Geometry: final body of the model. Coordinates: model frame, mm. A direction names the side the tool comes from. Give positions to 0.01 mm unless a question says otherwise; leave off trailing zeros. Order: outer loops, then holes, each group sorted by start corner. A loop starts at its lowest first (then second) coordinate and runs counter-clockwise, first axis right, second up. Notation, with made-up numbers: (56.5, 7) -> (82.5, 7) arc R12 ccw to (82.5, 13) -> close; hole circle Ø10 at (-28, 1). An arc over 180 degrees is marked (long way). Answer in a Markdown table with one row per item. Add a question column.
Q1. Set-up query: faces 4 (the face through (3, 0, 0)), 5 (the face through (3.5, 0, 43)), 6 (the face through (4.5, 7, 175)). Return all of +Z, -Z, +X, -X, +Y, -Y with unobstructed straight access to the full face (end or side cutting, diameter ignored); none if empty.
Q2. Pull-direction query (Y, two-part tool) for faces 1 (the face through (4.5, -7, 175)), 2 (the face through (1, 10, 174)), 3 (the face through (3.5, -2, 5)); classes: +Y half, -Y half, draft (parallel to the pull), parting line (faces both ways), or undercut.
Q3. Cut plane A-A on z = 94. Return the cut outline in (x, y).
Q4. Line query: line 1 along Y through (x, z) = (2.6, 225); line 2 along Z through (x, y) = (3.5, 6.5); line 3 along Y through (x, z) = (5.55, 225). Output: solid intervals per line, ascending. Write a range as from..to.
Q5. Contact query for flat-ended pins moving along their axis: P1, Ø2, axis at x = 3, y = 0.5, coming from the -Z side; P2, Ø1.8, axis at y = -1, z = 66, coming from the -X side; P3, Ø3, axis at y = -7.5, z = 179.45, coming from the -X side; P4, Ø10, axis at y = -1.5, z = 214, coming from the -X side. Output: stop coordinate, or through.
from build123d import *

# Parameters (mm, degrees)
SKETCH046_W             = 9
SKETCH046_H             = 250
PAD023_DEPTH            = 6.5
SKETCH043_R             = 1.75
POCKET019_DEPTH         = 6.5
LINEARPATTERN010_COUNT  = 13
LINEARPATTERN010_PITCH  = 20
SKETCH045_R             = 3
POCKET020_DEPTH         = 3.5
LINEARPATTERN011_COUNT  = 13
LINEARPATTERN011_PITCH  = 20
SKETCH044_W             = 20
SKETCH044_H             = 28.9
SKETCH044_R             = 1.75
PAD024_DEPTH            = 8
BODY010_ROLL_ANGLE      = 90
BODY010_PLACEMENT_ANGLE = -90


with BuildPart() as part:
    # Sketch046 → Pad023 (new body)
    with BuildSketch(Plane.XY):
        with Locations((0, 125)):
            Rectangle(SKETCH046_W, SKETCH046_H)
    extrude(amount=-PAD023_DEPTH)

    # Sketch043 → Pocket019 (cut)
    with BuildSketch(Plane.XY):
        with Locations((0, 5)):
            Circle(SKETCH043_R)
    pocket019 = extrude(amount=-POCKET019_DEPTH, mode=Mode.SUBTRACT)

    # LinearPattern010: Pocket019 ×13
    with Locations(*[(0, i * LINEARPATTERN010_PITCH, 0) for i in range(1, LINEARPATTERN010_COUNT)]):
        add(pocket019, mode=Mode.SUBTRACT)

    # Sketch045 → Pocket020 (cut)
    with BuildSketch(Plane.XY):
        with Locations((0, 5)):
            Circle(SKETCH045_R)
    pocket020 = extrude(amount=-POCKET020_DEPTH, mode=Mode.SUBTRACT)

    # LinearPattern011: Pocket020 ×13
    with Locations(*[(0, i * LINEARPATTERN011_PITCH, 0) for i in range(1, LINEARPATTERN011_COUNT)]):
        add(pocket020, mode=Mode.SUBTRACT)

    # Sketch044 → Pad024 (join)
    with BuildSketch(Plane.XY.offset(-4.5)):
        with Locations((0, 174.45)):
            Rectangle(SKETCH044_W, SKETCH044_H)
        with Locations((-7.5, 179.45)):
            Circle(SKETCH044_R, mode=Mode.SUBTRACT)
        with Locations((7.5, 179.45)):
            Circle(SKETCH044_R, mode=Mode.SUBTRACT)
        with Locations((7.5, 169.45)):
            Circle(SKETCH044_R, mode=Mode.SUBTRACT)
        with Locations((-7.5, 169.45)):
            Circle(SKETCH044_R, mode=Mode.SUBTRACT)
    extrude(amount=PAD024_DEPTH)


with BuildPart() as part_1:
    # Body010 roll: moved
    add(part.part.rotate(Axis((0, 0, 0), (1, 0, 0)), BODY010_ROLL_ANGLE))


with BuildPart() as part_2:
    # Body010 placement: moved
    add(part_1.part.rotate(Axis((0, 0, 0), (0, 0, 1)), BODY010_PLACEMENT_ANGLE))


solid = part_2.part
Completed:
| question | item | result |
|---|---|---|
| 1 | face 4 | -Z, +X, -X, +Y, -Y |
| 1 | face 5 | -X |
| 1 | face 6 | +Z, -Z, +X, +Y |
| 2 | face 1 | draft |
| 2 | face 2 | +Y half |
| 2 | face 3 | undercut |
| 3 | outline | (0, -4.5) -> (6.5, -4.5) -> (6.5, 4.5) -> (0, 4.5) -> close |
| 4 | line 1 | y = -4.5..-3, 3..4.5 |
| 4 | line 2 | z = 160..168.01, 170.89..178.01, 180.89..188.9 |
| 4 | line 3 | y = -4.5..-1.75, 1.75..4.5 |
| 5 | P1 | stops at z = 0 |
| 5 | P2 | stops at x = 3.5 |
| 5 | P3 | passes through |
| 5 | P4 | stops at x = 0 |
